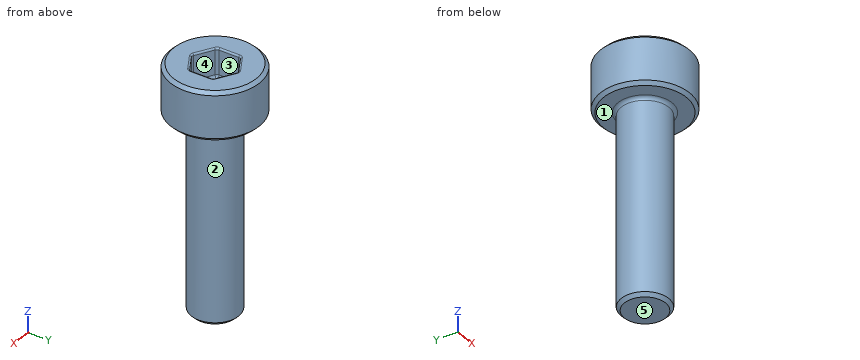
```python
from build123d import *

# Parameters (mm, degrees)
SCHNITT_LINEAR_AUSTRAGEN1_DEPTH = 1.8
FASE1_SIZE                      = 0.2
VERRUNDUNG1_R                   = 0.2
VERRUNDUNG2_R                   = 0.1


with BuildPart() as part:
    # Skizze1 → Rotation1 (revolve)
    with BuildSketch(Plane(origin=(0, 0, 0), x_dir=(0, 0, -1), z_dir=(1, 0, 0))):
        Polygon((-3, 0), (-3, 2.75), (0, 2.75), (0, 1.465), (12, 1.465), (12, 0), align=None)
    revolve(axis=Axis((0, 0, 21.919879518), (0, 0, -1)))

    # Skizze2 → Schnitt-Linear austragen1 (cut)
    with BuildSketch(Plane.XY.offset(3)):
        Polygon((1.25, -0.721687836), (1.25, 0.721687836), (0, 1.443375673), (-1.25, 0.721687836), (-1.25, -0.721687836), (0, -1.443375673), align=None)
    extrude(amount=-SCHNITT_LINEAR_AUSTRAGEN1_DEPTH, mode=Mode.SUBTRACT)

    # Fase1
    fase1_edges = [part.edges().sort_by_distance(p)[0] for p in [
        (0, -1.465, -12),
        (0, -2.75, 0),
        (0, -2.75, 3),
    ]]
    chamfer(fase1_edges, length=FASE1_SIZE)

    # Verrundung1
    verrundung1_edges = [part.edges().sort_by_distance(p)[0] for p in [
        (0.625, -1.082531755, 1.2),
        (1.25, -0.721687836, 2.1),
        (-0.625, -1.082531755, 1.2),
        (0, -1.443375673, 2.1),
        (-1.25, 0, 1.2),
        (-1.25, -0.721687836, 2.1),
        (-0.625, 1.082531755, 1.2),
        (-1.25, 0.721687836, 2.1),
        (0.625, 1.082531755, 1.2),
        (0, 1.443375673, 2.1),
        (1.25, 0, 1.2),
        (1.25, 0.721687836, 2.1),
        (0, -1.465, 0),
    ]]
    fillet(verrundung1_edges, radius=VERRUNDUNG1_R)

    # Verrundung2
    verrundung2_edges = [part.edges().sort_by_distance(p)[0] for p in [
        (-0.625, -1.082531755, 3),
        (-1.25, 0, 3),
        (-0.625, 1.082531755, 3),
        (0.625, 1.082531755, 3),
        (1.25, 0, 3),
        (0.625, -1.082531755, 3),
        (-1.223205081, -0.706217783, 3),
        (0, -1.412435565, 3),
        (1.223205081, -0.706217783, 3),
        (1.223205081, 0.706217783, 3),
        (0, 1.412435565, 3),
        (-1.223205081, 0.706217783, 3),
    ]]
    fillet(verrundung2_edges, radius=VERRUNDUNG2_R)


solid = part.part
```
Geometry: final body of the model. Coordinates: model frame, mm. Face numbers are marked on the shaded views. A direction names the side the tool comes from. Give positions to 0.01 mm unless a question says otherwise; leave off trailing zeros. Write each loop counter-clockwise with the first axis right and the second up, starting at its lowest first coordinate (ties: lowest second). Pieces come first, ordered by that corner, then holes.
1. Section query C-C, the plane z = -9.75. Return loops of the section in (x, y) (3 decimals).
2. Section query B-B, the plane y = 0. Return loops of the section in (x, z) (3 decimals), then the cut area to 3 significant figures.
3. Pin query (flat end, axial travel): P1, Ø1.5, axis at y = 1, z = -2, coming from the +X side; P2, Ø2, axis at x = -2, z = -9.5, coming from the -Y side. Return the tip coordinate at first contact, or that it passes through.
4. Reachability of the marked faces 4 and 5 from +Z, -Z, +X, -X, +Y, -Y: full face, straight path, thin tool, end or side. Return the list, or none.
5. Line query: probe 1 along Y at (x, z) = (-0.4, -2); probe 2 along Z at (x, y) = (1.7, 0.3); probe 3 along Y at (x, z) = (-0.3, 1.5). Output: solid intervals per line, ascending.
6. Draft query along Y for the marked faces 1, 2 and 3. Return one class per face: released by +Y, released by -Y, zero draft, split by the parting line, or undercut.
7. Section query A-A, the plane z = 2. Return loops of the section in (x, y), then the cut area to 3 significant figures.
Computed:
1. outline: circle Ø2.93 at (0, 0)
2. outline: (-2.75, 0.2) - (-2.55, 0) - (-1.665, 0) arc R0.2 cw to (-1.465, -0.2) - (-1.465, -11.8) - (-1.265, -12) - (1.265, -12) - (1.465, -11.8) - (1.465, -0.2) arc R0.2 cw to (1.665, 0) - (2.55, 0) - (2.75, 0.2) - (2.75, 2.8) - (2.55, 3) - (1.35, 3) arc R0.1 ccw to (1.25, 2.9) - (1.25, 1.4) arc R0.2 cw to (1.05, 1.2) - (-1.05, 1.2) arc R0.2 cw to (-1.25, 1.4) - (-1.25, 2.9) arc R0.1 ccw to (-1.35, 3) - (-2.55, 3) - (-2.75, 2.8) - close
2. area: 47.1 mm2
3. P1: stops at x = 1.44
3. P2: stops at y = -1.07
4. face 4: +Z
4. face 5: -Z, +X, -X, +Y, -Y
5. probe 1: y = -1.41 to 1.41
5. probe 2: z = 0 to 3
5. probe 3: y = -2.73 to -1.27, 1.27 to 2.73
6. face 1: zero draft
6. face 2: split by the parting line
6. face 3: undercut
7. outline: circle Ø5.5 at (0, 0); hole (-1.25, -0.61) arc R0.2 ccw to (-1.15, -0.78) - (-0.1, -1.39) arc R0.2 ccw to (0.1, -1.39) - (1.15, -0.78) arc R0.2 ccw to (1.25, -0.61) - (1.25, 0.61) arc R0.2 ccw to (1.15, 0.78) - (0.1, 1.39) arc R0.2 ccw to (-0.1, 1.39) - (-1.15, 0.78) arc R0.2 ccw to (-1.25, 0.61) - close
7. area: 18.4 mm2
